The model under review builds one solid part; all positions refer to its coordinate system, in mm. Face numbers are marked on the shaded views. A direction names the side the tool comes from. Give positions to 0.01 mm unless a question says otherwise; leave off trailing zeros. Order: outer loops, then holes, each group sorted by start corner. A loop starts at its lowest first (then second) coordinate and runs counter-clockwise, first axis right, second up. Notation, with made-up numbers: (87.5, 31.5) - (115.5, 31.5) arc R13 cw to (115.5, 40.5) - close; hole circle Ø11 at (84, 23). An arc over 180 degrees is marked (long way). Write item = value, one per line. Start each with the question number.
1. We need section A-A, the plane y = 12.7. Give the boundary of the cut face in (x, z) (3 decimals), and give its area (3 significant figures).
2. For P1, Ø3, axis at x = 32.5, y = 26.5, coming from the -Z side; P2, Ø2, axis at x = 13.5, z = 34, coming from the -Y side; P3, Ø4, axis at x = 29.5, y = 9, coming from the +Z side (3 decimals), all flat-tipped, find the tip position at first contact; note any pin that passes through.
3. We need section D-D, the plane z = 6. Give the boundary of the cut face in (x, y) (3 decimals).
4. Machinability: for the marked faces 1 and 2, which of the approach directions +Z, -Z, +X, -X, +Y, -Y give a long, thin tool a straight path to every point of the face, cutting with its end or side? Answer none if there is none.
5. Wall thickness on probe 1 along Y at (x, z) = (27, 31.5) (3 decimals); probe 2 along Z at (x, y) = (6.5, 4) (3 decimals): over which ranges is each line inside the solid? List them lowest first.
6. We need section B-B, the plane x = 6.35. Give the boundary of the cut face in (y, z) (3 decimals).
7. We need section C-C, the plane x = 13. Give the boundary of the cut face in (y, z) (3 decimals), and give its area (3 significant figures).
Autodesk Inventor part; units mm, degrees
ref_plane "YZ Plane" through (0, 0, 0) normal (1, 0, 0) x (0, 1, 0)
ref_plane "XZ Plane" through (0, 0, 0) normal (0, 1, 0) x (-1, 0, 0)
ref_plane "XY Plane" through (0, 0, 0) normal (0, 0, 1) x (1, 0, 0)
sketch "Sketch1" plane through (0, 0, 0) normal (0, 0, 1) x (1, 0, 0)
  line L0 (0, 0) -> (38.1, 0)
  line L1 (38.1, 0) -> (38.1, 25.4)
  line L2 (38.1, 25.4) -> (0, 25.4)
  line L3 (0, 25.4) -> (0, 0)
  circle A0 centre (6.35, 12.7) radius 2.0701
  circle A1 centre (31.75, 12.7) radius 2.0701
  dimension "d0" = 38.1
  dimension "d1" = 25.4
  dimension "d2" = 4.1402
  dimension "d3" = 12.7
  dimension "d4" = 6.35
  dimension "d7" = 25.4
extrude "Plate1" add sketch "Sketch1" along normal blind 3.175
sketch "Sketch2" plane through (0, 26.67, 4.445) normal (0, 1, 0) x (-1, 0, 0)
  line L0 (-38.1, 0) -> (0, 0)
  line L1 (0, 0) -> (0, 46.355)
  line L2 (0, 46.355) -> (-38.1, 46.355)
  line L3 (-38.1, 46.355) -> (-38.1, 0)
edge flange "Flange1" height 50.8 angle 90 thickness 3.175 bend radius 1.27 thickness toward (0, 1, 0) relief tear relief width 3.175 relief depth 1.5875 edges at (19.05, 25.4, 3.175) wall of the first edge with corners at (38.1, 26.67, 4.445) (0, 26.67, 4.445) (0, 26.67, 50.8) (38.1, 26.67, 50.8)
bend "Bend1"
corner "Corner1"
sketch "Sketch3" plane through (0, 29.845, 50.8) normal (0, 1, 0) x (1, 0, 0)
  line L0 (38.1, 46.355) -> (0, 46.355)
  line L1 (32.3088, 33.655) -> (13.2588, 33.655) construction
  line L2 (13.2588, 33.655) -> (13.2588, 0.381) construction
  line L3 (13.2588, 0.381) -> (32.3088, 0.381) construction
  line L4 (32.3088, 0.381) -> (32.3088, 33.655) construction
  line L5 (32.3088, 5.969) -> (13.2588, 5.969) construction
  circle A0 centre (29.1338, 5.969) radius 2.413
  line L6 (22.7838, 0.381) -> (22.7838, 33.655) construction
  circle A1 centre (16.4338, 5.969) radius 2.413
  line L7 (32.3088, 17.018) -> (13.2588, 17.018) construction
  circle A2 centre (29.1338, 28.067) radius 2.413
  circle A3 centre (16.4338, 28.067) radius 2.413
  line L8 (0, 0) -> (0, 46.355)
  point P0 (0, 50.8)
  dimension "d23" = 19.05
  dimension "d24" = 33.274
  dimension "d25" = 5.588
  dimension "d26" = 3.175
  dimension "d27" = 4.826
  dimension "d29" = 12.7
  dimension "d32" = 13.2588
extrude "Cut1" cut sketch "Sketch3" against normal blind 3.175
equation "\"d30\" = Thickness"
equation "\"d13\" = BendReliefWidth"
equation "\"d14\" = BendReliefDepth"
equation "\"d15\" = MinimumRemnant"
equation "\"d16\" = BendRadius"
equation "\"d20\" = CornerReliefSize"
equation "\"d21\" = GapSize"
equation "\"d22\" = JacobiRadiusSize"
equation "\"BendRadius\" = Thickness"
equation "\"BendReliefWidth\" = Thickness"
equation "\"BendReliefDepth\" = 0.5 * Thickness"
equation "\"CornerReliefSize\" = 4 * Thickness"
equation "\"MinimumRemnant\" = 2 * Thickness"
equation "\"TransitionRadius\" = BendRadius"
equation "\"JacobiRadiusSize\" = BendRadius"
equation "\"GapSize\" = Thickness"
equation "\"d12\" = BendRadius"
properties part number "Pneumatic Piston Back Flange (Left Custom)" material "Aluminum 6061"
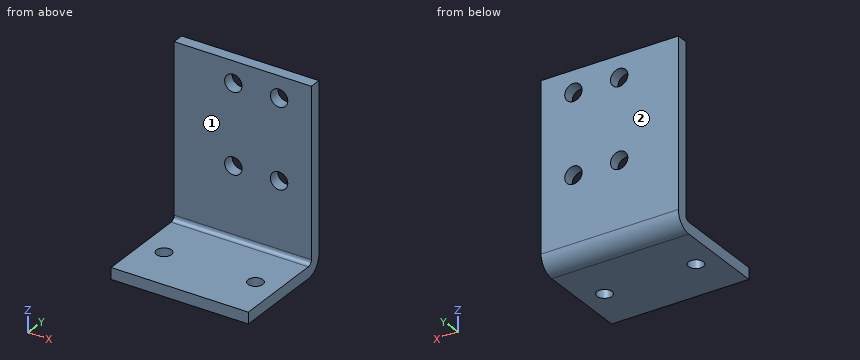
Model answer:
q1.outline = (0, 0) - (4.28, 0) - (4.28, 3.175) - (0, 3.175) - close; (8.42, 0) - (29.68, 0) - (29.68, 3.175) - (8.42, 3.175) - close; (33.82, 0) - (38.1, 0) - (38.1, 3.175) - (33.82, 3.175) - close
q1.area = 94.7 mm2
q2.P1 = 0
q2.P2 = 26.67
q2.P3 = 3.175
q3.outline = (0, 26.67) - (38.1, 26.67) - (38.1, 29.845) - (0, 29.845) - close
q4.face_1 = +Z, +X, -X, -Y
q4.face_2 = +Z, -Z, +X, -X, +Y
q5.probe_1 = 26.67 to 29.845
q5.probe_2 = 0 to 3.175
q6.outline = (0, 0) - (10.63, 0) - (10.63, 3.175) - (0, 3.175) - close; (14.77, 0) - (25.4, 0) arc R4.445 ccw to (29.845, 4.445) - (29.845, 50.8) - (26.67, 50.8) - (26.67, 4.445) arc R1.27 cw to (25.4, 3.175) - (14.77, 3.175) - close
q7.outline = (0, 0) - (25.4, 0) arc R4.445 ccw to (29.845, 4.445) - (29.845, 50.8) - (26.67, 50.8) - (26.67, 4.445) arc R1.27 cw to (25.4, 3.175) - (0, 3.175) - close
q7.area = 242 mm2
